Source: three-view drawing plus pictorial views. Frame: mm from the lowest corner of the part. A direction names the side the tool comes from. Coordinates: 2 decimals unless noted, no trailing zeros. Order: outer loops, then holes, each group sorted by start corner. A loop starts at its lowest first (then second) coordinate and runs counter-clockwise, first axis right, second up. Notation, with made-up numbers: (17, 43.5) -> (76, 43.5) arc R13 ccw to (76, 62.5) -> close; hole circle Ø3 at (51.5, 69). An arc over 180 degrees is marked (long way). Use CSV: the item, a comma, the result in double quotes. Start each with the question number.
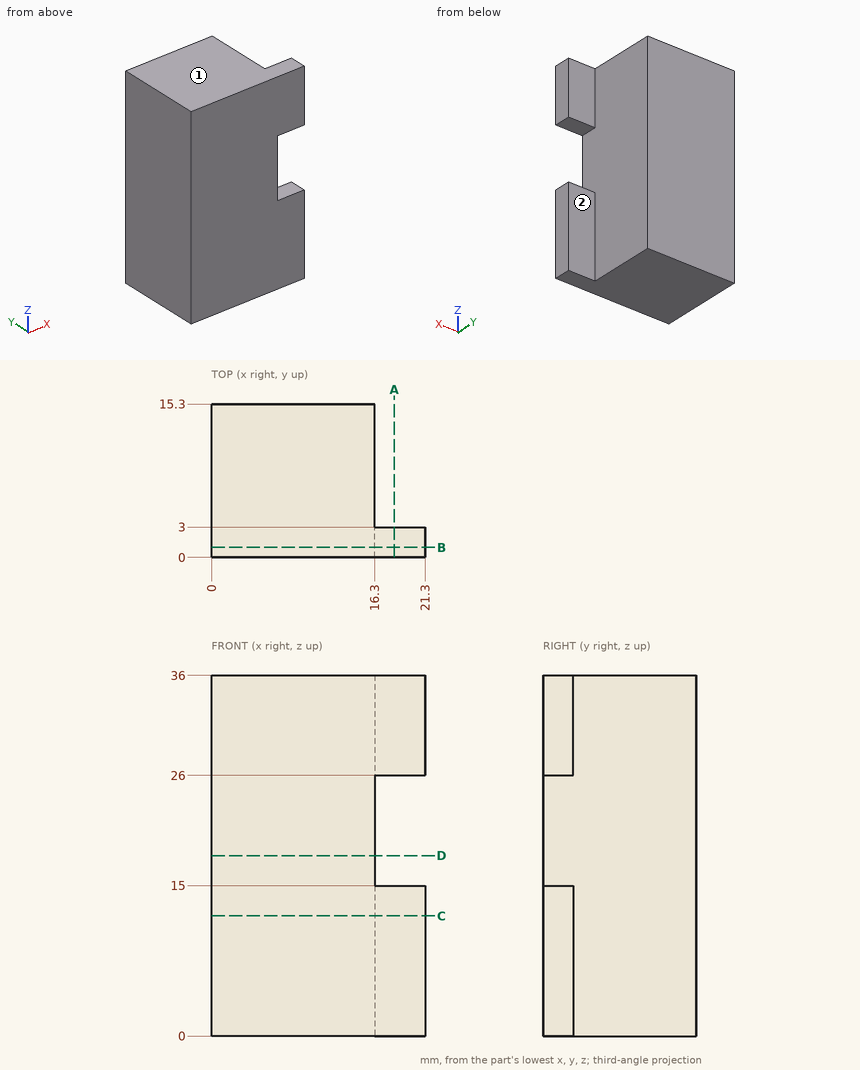
1. Contact query for flat-ended pins moving along their axis: P1, Ø2.5, axis at x = 19.5, z = 7, coming from the +Y side; P2, Ø2, axis at y = 12.5, z = 30.5, coming from the +X side; P3, Ø3, axis at x = 3, z = 27.5, coming from the -Y side. Output: stop coordinate, or through.
2. Section D-D on z = 18. Return loops of the section in (x, y).
3. Material intervals for line 1 along Z through (x, y) = (18, 2.5); line 2 along X through (y, z) = (14, 2); line 3 along Y through (x, z) = (19.25, 8), sorted ascending.
4. Section C-C on z = 12. Return loops of the section in (x, y).
5. Section B-B on y = 1. Return loops of the section in (x, z), then the cut area to 3 significant figures.
6. Section A-A on x = 18.25. Return loops of the section in (y, z), then the cut area to 3 significant figures.
7. Access query for the marked faces 1 and 2. Directions: +Z, -Z, +X, -X, +Y, -Y. A direction counts if a zero-diameter tool reaches every point of the face in a straight line with its end or side. Return the directions, or none.
Values follow:
1,P1,"stops at y = 3"
1,P2,"stops at x = 16.3"
1,P3,"stops at y = 0"
2,outline,"(0, 0) -> (16.3, 0) -> (16.3, 15.3) -> (0, 15.3) -> close"
3,line 1,"z = 0 to 15, 26 to 36"
3,line 2,"x = 0 to 16.3"
3,line 3,"y = 0 to 3"
4,outline,"(0, 0) -> (21.3, 0) -> (21.3, 3) -> (16.3, 3) -> (16.3, 15.3) -> (0, 15.3) -> close"
5,outline,"(0, 0) -> (21.3, 0) -> (21.3, 15) -> (16.3, 15) -> (16.3, 26) -> (21.3, 26) -> (21.3, 36) -> (0, 36) -> close"
5,area,"712 mm2"
6,outline,"(0, 0) -> (3, 0) -> (3, 15) -> (0, 15) -> close; (0, 26) -> (3, 26) -> (3, 36) -> (0, 36) -> close"
6,area,"75.0 mm2"
7,face 1,"+Z, +X, -X, +Y, -Y"
7,face 2,"+Z, -Z, +X, +Y"
